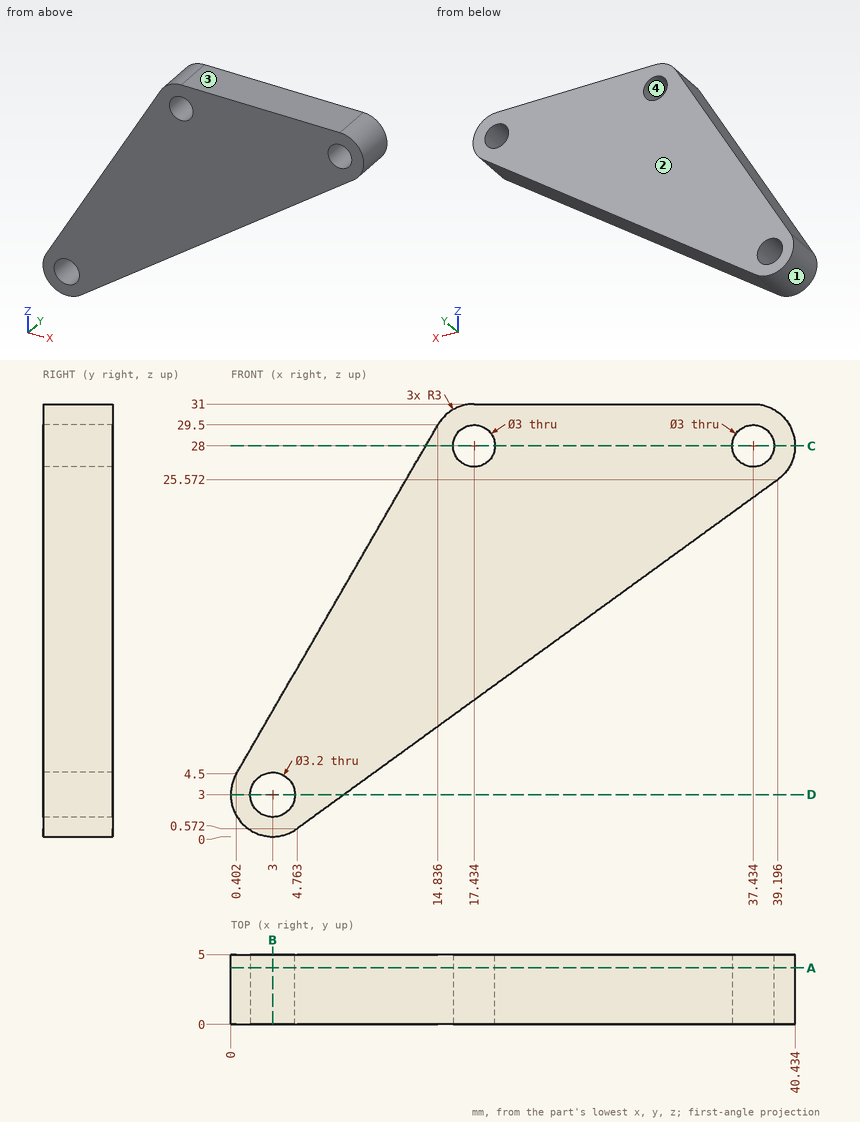
Input: dimensioned drawing with shaded views. Units: mm. Origin: part minimum x, y, z. Coordinates: 2 decimals unless noted, no trailing zeros. Order: outer loops, then holes, each group sorted by start corner. A loop starts at its lowest first (then second) coordinate and runs counter-clockwise, first axis right, second up.
(1) Section query C-C (z = 28). Return the cut outline in (x, y).
(2) Material intervals for probe 1 along X at (y, z) = (2, 2.5) (1 decimal); probe 2 along Z at (x, y) = (3, 3.35); probe 3 along Z at (x, y) = (2.5, 3.45) (1 decimal), sorted ascending.
(3) Draft query along Z for the marked faces 1, 2, 3 and 4. Return one class per face: pulls with the +Z half, pulls with the -Z half, needs draft (parallel to the pull), parting line crosses it, or undercut.
(4) Section query A-A (y = 4.05). Return the cut outline in (x, z) (1 decimal).
(5) First-contact query: pin 1 (2.5 mm diameter, centred on x = 37.43, z = 28, fed in from -Y); pin 2 (3 mm diameter, centred on x = 13.5, y = 4.5, fed in from +Z) (1 decimal). Flat tips, straight axial feed; report the tip coordinate or a pass-through.
(6) Section query B-B (x = 3). Return the cut outline in (y, z).
(7) Section query D-D (z = 3). Return the cut outline in (x, y).
Solution:
1. outline: (13.97, 0) - (15.93, 0) - (15.93, 5) - (13.97, 5) - close; (18.93, 0) - (35.93, 0) - (35.93, 5) - (18.93, 5) - close; (38.93, 0) - (40.43, 0) - (40.43, 5) - (38.93, 5) - close
2. probe 1: x = 0 to 1.5, 4.5 to 7.4
2. probe 2: z = 0 to 1.4, 4.6 to 9
2. probe 3: z = 0 to 1.5, 4.5 to 8.1
3. face 1: parting line crosses it
3. face 2: needs draft
3. face 3: pulls with the +Z half
3. face 4: undercut
4. outline: (0.4, 4.5) arc R3 ccw to (4.8, 0.6) - (39.2, 25.6) arc R3 ccw to (37.4, 31) - (17.4, 31) arc R3 ccw to (14.8, 29.5) - close; hole circle Ø3.2 at (3, 3); hole circle Ø3 at (17.4, 28); hole circle Ø3 at (37.4, 28)
5. pin 1: passes through
5. pin 2: stops at z = 29.8
6. outline: (0, 0) - (5, 0) - (5, 1.4) - (0, 1.4) - close; (0, 4.6) - (5, 4.6) - (5, 9) - (0, 9) - close
7. outline: (0, 0) - (1.4, 0) - (1.4, 5) - (0, 5) - close; (4.6, 0) - (8.11, 0) - (8.11, 5) - (4.6, 5) - close
